from build123d import *

# Parameters (mm, degrees)
SKETCH1_W           = 35.5
SKETCH1_H           = 19.55
BOSS_EXTRUDE1_DEPTH = 1.2
SKETCH2_W           = 35.5
SKETCH2_H           = 1
BOSS_EXTRUDE2_DEPTH = 7.5
FILLET1_R           = 1
SKETCH3_W           = 1
SKETCH3_H           = 6
BOSS_EXTRUDE3_DEPTH = 1.3
FILLET2_R           = 0.6
FILLET3_R           = 1.6


with BuildPart() as part:
    # Sketch1 → Boss-Extrude1 (new body)
    with BuildSketch(Plane.XY):
        Rectangle(SKETCH1_W, SKETCH1_H)
    extrude(amount=BOSS_EXTRUDE1_DEPTH)

    # Sketch2 → Boss-Extrude2 (add)
    with BuildSketch(Plane(origin=(0, 0, 0), x_dir=(-1, 0, 0), z_dir=(0, 0, -1))):
        with Locations((0, 9.275)):
            Rectangle(SKETCH2_W, SKETCH2_H)
        with Locations((0, -9.275)):
            Rectangle(SKETCH2_W, SKETCH2_H)
    extrude(amount=BOSS_EXTRUDE2_DEPTH)

    # Fillet1
    fillet1_edges = [part.edges().sort_by_distance(p)[0] for p in [
        (0, 8.775, 0),
        (0, -8.775, 0),
    ]]
    fillet(fillet1_edges, radius=FILLET1_R)

    # Sketch3 → Boss-Extrude3 (add)
    with BuildSketch(Plane(origin=(0, 0, 0), x_dir=(-1, 0, 0), z_dir=(0, 0, -1))):
        with Locations((17.25, 0)):
            Rectangle(SKETCH3_W, SKETCH3_H)
        with Locations((-17.25, 0)):
            Rectangle(SKETCH3_W, SKETCH3_H)
    extrude(amount=BOSS_EXTRUDE3_DEPTH)

    # Fillet2
    fillet2_edges = [part.edges().sort_by_distance(p)[0] for p in [
        (-17.25, 3, 0),
        (-17.25, -3, 0),
        (-17.25, 3, -1.3),
        (-17.25, -3, -1.3),
        (17.25, 3, 0),
        (17.25, -3, 0),
        (17.25, 3, -1.3),
        (17.25, -3, -1.3),
    ]]
    fillet(fillet2_edges, radius=FILLET2_R)

    # Fillet3
    fillet3_edges = [part.edges().sort_by_distance(p)[0] for p in [
        (17.75, 9.275, -7.5),
        (-17.75, 9.275, -7.5),
        (17.75, -9.275, -7.5),
        (-17.75, -9.275, -7.5),
    ]]
    fillet(fillet3_edges, radius=FILLET3_R)


solid = part.part
For this review, take the finished solid that the model builds, in its own axes (mm). A direction names the side the tool comes from. Give positions to 0.01 mm unless a question says otherwise; leave off trailing zeros. Loops run counter-clockwise (first coordinate to the right, second up) from the corner with the lowest first, then second, coordinate; pieces in that order, holes last. Notation, with made-up numbers: (74, -0.5) -> (91, -0.5) arc R16 cw to (91, 27.5) -> close; hole circle Ø3 at (89, 45). An arc over 180 degrees is marked (long way). One line per question, with ' | ' between items.
1) For faces 4 (the flat face through (0, 8.775, -4)), 5 (the cylindrical face through (17.29, 9.28, -7.02)), 6 (the flat face through (16.75, 0, -1)), list the 3-axis set-ups (+Z, -Z, +X, -X, +Y, -Y) from which the entire face can be reached by the end or side of a thin tool; tool diameter is ignored.
Resolved:
face 4: -Z, +X, -X | face 5: -Z, +X, +Y, -Y | face 6: -Z
2) To check wall thickness, follow probe 1 along Y at (x, z) = (5.5, -2) (3 decimals); probe 2 along Z at (x, y) = (-5, 5.25); probe 3 along Y at (x, z) = (14, -0.25) (3 decimals). State the ranges of each line that lie inside material, in increasing order.
Resolved:
probe 1: y = -9.775 to -8.775, 8.775 to 9.775 | probe 2: z = 0 to 1.2 | probe 3: y = -9.775 to -8.436, 8.436 to 9.775
3) We need section B-B (x = 0). Write out the cut boundary in (y, z) (3 decimals), plus the area to 3 significant figures.
Resolved:
outline: (-9.775, -7.5) -> (-8.775, -7.5) -> (-8.775, -1) arc R1 cw to (-7.775, 0) -> (7.775, 0) arc R1 cw to (8.775, -1) -> (8.775, -7.5) -> (9.775, -7.5) -> (9.775, 1.2) -> (-9.775, 1.2) -> close | area: 38.9 mm2
4) Insertion check: pin 1 Ø1.1 at (x, y) = (17, 1) entering from -Z; pin 2 Ø4 at (x, y) = (9, -8) entering from -Z; pin 3 Ø10 at (x, y) = (-2, -3) entering from -Z. Each pin has a flat end and moves straight along its axis. Give the tip position at first contact, or say it passes through.
Resolved:
pin 1: stops at z = -1.3 | pin 2: stops at z = -7.5 | pin 3: stops at z = -0.03
5) We need section A-A (z = -5). Write out the cut boundary in (x, y) (3 decimals).
Resolved:
outline: (-17.75, -9.775) -> (17.75, -9.775) -> (17.75, -8.775) -> (-17.75, -8.775) -> close; (-17.75, 8.775) -> (17.75, 8.775) -> (17.75, 9.775) -> (-17.75, 9.775) -> close
6) We need section C-C (y = -2). Write out the cut boundary in (x, z), plus the area to 3 significant figures.
Resolved:
outline: (-17.75, -1.3) -> (-16.75, -1.3) -> (-16.75, 0) -> (16.75, 0) -> (16.75, -1.3) -> (17.75, -1.3) -> (17.75, 1.2) -> (-17.75, 1.2) -> close | area: 45.2 mm2
7) We need section D-D (y = -4.5). Write out the cut boundary in (x, z), plus the area to 3 significant figures.
Resolved:
outline: (-17.75, 0) -> (17.75, 0) -> (17.75, 1.2) -> (-17.75, 1.2) -> close | area: 42.6 mm2
8) The part is to be moulded in two halves that separate along X. For faces 1 (the flat face through (0, 0, 0)), 2 (the cylindrical face through (-17.29, 9.28, -7.02)), 3 (the flat face through (0, -9, -7.5)), say which applies: +X half, -X half, draft (parallel to the pull), parting line (faces both ways), or undercut.
Resolved:
face 1: undercut | face 2: -X half | face 3: draft
